```python
from build123d import *


with BuildPart() as f1:
    # F0 (on Front) → F1 (revolve)
    with BuildSketch(Plane.XZ):
        with BuildLine():
            Line((37.5, 6.25), (0, 6.25))
            Line((0, 6.25), (-37.5, 6.25))
            ThreePointArc((-37.5, 6.25), (-42.082891, 7.361968), (-45.646576, 10.450578))
            Line((-45.646576, 10.450578), (-59.267242, 10.450578))
            Line((-59.267242, 10.450578), (-59.267242, 0))
            Line((-59.267242, 0), (0, 0))
            Line((0, 0), (59.267242, 0))
            Line((59.267242, 0), (59.267242, 10.450578))
            Line((59.267242, 10.450578), (45.646576, 10.450578))
            ThreePointArc((45.646576, 10.450578), (42.082891, 7.361968), (37.5, 6.25))
        make_face()
    revolve(axis=Axis((-29.633621, 0, 0), (1, 0, 0)))


solid = f1.part
```
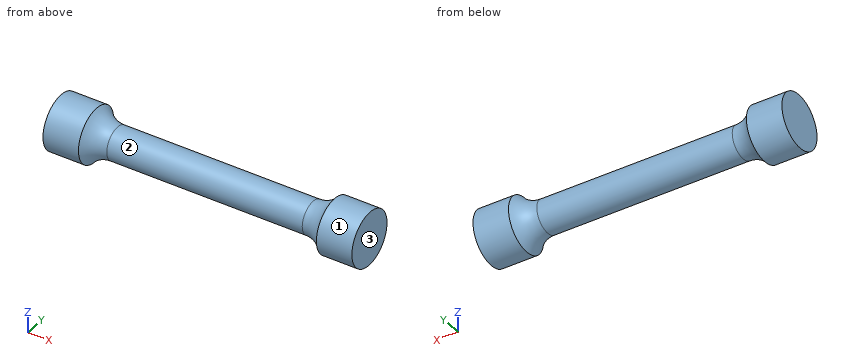
Verification items for the finished model (mm, model axes). Face numbers are marked on the shaded views. Coordinates: 2 decimals unless noted, no trailing zeros. Loops run counter-clockwise (first coordinate to the right, second up) from the corner with the lowest first, then second, coordinate; pieces in that order, holes last. Notation, with made-up numbers: (-23, 85.5) - (8, 85.5) arc R20 cw to (8, 120.5) - close; hole circle Ø3 at (60, 88.5). An arc over 180 degrees is marked (long way). Return JSON: item names as keys, results as strings.
1. Go/stop test with flat-tipped pins: pin 1 (2 mm diameter, centred on x = -0.5, z = -4, fed in from -Y); pin 2 (1 mm diameter, centred on x = 47, y = -4, fed in from -Z); pin 3 (2 mm diameter, centred on x = -46.5, z = -8, fed in from +Y). Record where each tip stops, or that it passes through.
Established:
{"pin 1": "stops at y = -5.48", "pin 2": "stops at z = -9.85", "pin 3": "stops at y = 7.76"}
2. Section check C-C, the plane x = -49.5. Record the boundary of the cut face in (y, z).
Established:
{"outline": "circle Ø20.9 at (0, 0)"}
3. Mould release check, pull along X, two halves, no side actions. Record for the marked faces 1, 2 and 3: +X half, -X half, draft (parallel to the pull), parting line (faces both ways), or undercut.
Established:
{"face 1": "draft", "face 2": "undercut", "face 3": "+X half"}
4. Thickness scan on L1, parallel to X at y = -7, z = -5.75; L2, parallel to X at y = -1.5, z = 7.5; L3, parallel to Z at x = -7, y = 2.75. Record the ranges inside material, lowest first.
Established:
{"L1": "x = -59.27 to -44.45, 44.45 to 59.27", "L2": "x = -59.27 to -42.6, 42.6 to 59.27", "L3": "z = -5.61 to 5.61"}
5. Section check A-A, the plane z = 0. Record the boundary of the cut face in (x, y).
Established:
{"outline": "(-59.27, -10.45) - (-45.65, -10.45) arc R10 cw to (-37.5, -6.25) - (37.5, -6.25) arc R10 cw to (45.65, -10.45) - (59.27, -10.45) - (59.27, 10.45) - (45.65, 10.45) arc R10 cw to (37.5, 6.25) - (-37.5, 6.25) arc R10 cw to (-45.65, 10.45) - (-59.27, 10.45) - close"}
6. Section check D-D, the plane x = 6. Record the boundary of the cut face in (y, z).
Established:
{"outline": "circle Ø12.5 at (0, 0)"}
